The figure shows three views and two pictorial views of one solid part (mm, origin at its lowest corner). Answer the questions. Coordinates: 2 decimals unless noted, no trailing zeros. Write each loop counter-clockwise with the first axis right and the second up, starting at its lowest first coordinate (ties: lowest second). Pieces come first, ordered by that corner, then holes.
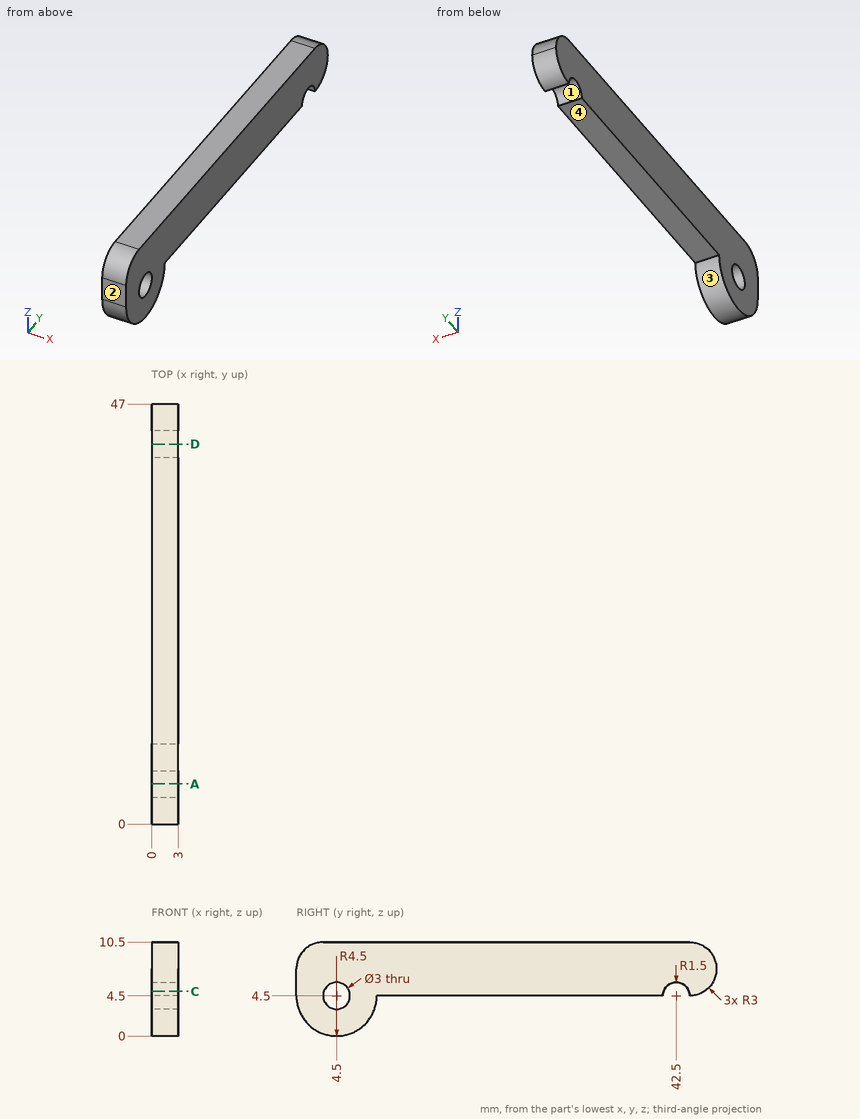
Q1. The part is cut by section C-C, the plane z = 5. Write down the section's boundary in (x, y).
Answers below:
outline: (0, 0) - (3, 0) - (3, 3.09) - (0, 3.09) - close; (0, 5.91) - (3, 5.91) - (3, 41.09) - (0, 41.09) - close; (0, 43.91) - (3, 43.91) - (3, 45.66) - (0, 45.66) - close
Q2. Find the intervals of material crossed by probe 1 along Y at (x, z) = (2.35, 3.5); probe 2 along Z at (x, y) = (0.2, 10.5); probe 3 along Y at (x, z) = (1.4, 4.75), in increasing order.
Answers below:
probe 1: y = 0.11 to 3.38, 5.62 to 8.89
probe 2: z = 4.5 to 10.5
probe 3: y = 0 to 3.02, 5.98 to 41.02, 43.98 to 45.2
Q3. The part is cut by section A-A, the plane y = 4.5. Write down the section's boundary in (x, z).
Answers below:
outline: (0, 0) - (3, 0) - (3, 3) - (0, 3) - close; (0, 6) - (3, 6) - (3, 10.5) - (0, 10.5) - close
Q4. Given pin 1 (0.9 mm diameter, centred on x = 1.5, y = 32.5, fed in from -Z), flat-ended and moving along its own axis, determine where the tip first touches the part or whether it passes through.
Answers below:
pin 1: stops at z = 4.5
Q5. The part is cut by section D-D, the plane y = 42.5. Write down the section's boundary in (x, z), then the cut area to 3 significant figures.
Answers below:
outline: (0, 6) - (3, 6) - (3, 10.5) - (0, 10.5) - close
area: 13.5 mm2
Q6. Determine the mould class of the marked faces 1, 2, 3 and 4 for opening direction Y: released by +Y, released by -Y, zero draft, split by the parting line, or undercut.
Answers below:
face 1: undercut
face 2: released by -Y
face 3: split by the parting line
face 4: zero draft
